```python
from build123d import *

# Parameters (mm, degrees)
SKETCH_1_R               = 2.5
EXTRUDE_1_DEPTH          = 2.5
CUT_EXTRUDE_1_REACH      = 65.602
SKETCH_2_R               = 2
PATTERN_CIRCULAR_1_COUNT = 6
FILLET_1_R               = 3


with BuildPart() as part:
    # 草圖1 → 填料-伸長1 (new, symmetric)
    with BuildSketch(Plane.XY):
        with BuildLine():
            Line((17.895530168, 10), (50, 10))
            ThreePointArc((50, 10), (60, 0), (50, -10))
            Line((50, -10), (17.895530168, -10))
            ThreePointArc((17.895530168, -10), (-20.5, 0), (17.895530168, 10))
        make_face()
        with Locations((50, 0)):
            Circle(SKETCH_1_R, mode=Mode.SUBTRACT)
    extrude(amount=EXTRUDE_1_DEPTH, both=True)

    # 草圖2 → 除料-伸長1 (cut, up to next)
    with BuildSketch(Plane.XY.offset(2.5), mode=Mode.PRIVATE) as cut_extrude_1_sk1:
        with Locations((0, 15.5)):
            Circle(SKETCH_2_R)
    cut_extrude_1_tool1 = extrude(cut_extrude_1_sk1.sketch, amount=-CUT_EXTRUDE_1_REACH, mode=Mode.PRIVATE) & part.part
    cut_extrude_1 = cut_extrude_1_tool1.solids().sort_by_distance((0, 15.5, 2.5))[0]
    add(cut_extrude_1, mode=Mode.SUBTRACT)

    # 環狀複製排列1: 除料-伸長1 ×6 about axis
    pattern_circular_1_axis = Axis((0, 0, 0), (0, 0, 1))
    for i in range(1, PATTERN_CIRCULAR_1_COUNT):
        add(cut_extrude_1.rotate(pattern_circular_1_axis, i * 360 / PATTERN_CIRCULAR_1_COUNT), mode=Mode.SUBTRACT)

    # 圓角1
    fillet_1_edges = [part.edges().sort_by_distance(p)[0] for p in [
        (17.895530168, 10, 0),
        (17.895530168, -10, 0),
    ]]
    fillet(fillet_1_edges, radius=FILLET_1_R)


solid = part.part
```
Verification items for the finished model (mm, model axes). A direction names the side the tool comes from. Round coordinates to 2 decimals unless told otherwise and drop trailing zeros. Write each loop counter-clockwise with the first axis right and the second up, starting at its lowest first coordinate (ties: lowest second). Pieces come first, ordered by that corner, then holes.
1. Section check B-B on x = 0. Enter the section's corners in (y, z).
2. Section check C-C on z = 0.65. Enter the section's corners in (x, y).
3. Draft check along Y on faces 1 (the cylindrical face through (52.31, -0.96, -0.04)), 2 (the cylindrical face through (18.141, -10.366, 0.035)), 3 (the cylindrical face through (60, 0, 0)). Enter one of: +Y half, -Y half, draft (parallel to the pull), parting line (faces both ways), or undercut.
4. Access from +Z, -Z, +X, -X, +Y, -Y to the whole of each face (thin tool, end or side, straight path). Record for faces 4 (the flat face through (35, -10, 0)), 5 (the cylindrical face through (-13.86, -9.7, 0.04)), 6 (the flat face through (35, 10, 0)).
5. Section check D-D on y = 7.75. Enter the section's corners in (x, z).
6. Scan lines: L1, parallel to Y at x = 0, z = 1.4; L2, parallel to X at y = 9, z = 1.8; L3, parallel to X at y = 8, z = -0.2. Record each from-to range of solid material in increasing order.
7. Section check A-A on y = 0. Enter the section's corners in (x, z).
Answer:
1. outline: (-20.5, -2.5) - (-17.5, -2.5) - (-17.5, 2.5) - (-20.5, 2.5) - close; (-13.5, -2.5) - (13.5, -2.5) - (13.5, 2.5) - (-13.5, 2.5) - close; (17.5, -2.5) - (20.5, -2.5) - (20.5, 2.5) - (17.5, 2.5) - close
2. outline: (17.08, -11.34) arc R3 cw to (19.58, -10) - (50, -10) arc R10 ccw to (50, 10) - (19.58, 10) arc R3 cw to (17.08, 11.34) arc R20.5 ccw (long way) to start; hole circle Ø4 at (-13.42, -7.75); hole circle Ø4 at (-13.42, 7.75); hole circle Ø4 at (0, -15.5); hole circle Ø4 at (0, 15.5); hole circle Ø4 at (13.42, -7.75); hole circle Ø4 at (13.42, 7.75); hole circle Ø5 at (50, 0)
3. face 1: undercut
3. face 2: -Y half
3. face 3: parting line
4. face 4: +Z, -Z, +X, -Y
4. face 5: +Z, -Z
4. face 6: +Z, -Z, +X, +Y
5. outline: (-18.98, -2.5) - (-15.42, -2.5) - (-15.42, 2.5) - (-18.98, 2.5) - close; (-11.42, -2.5) - (11.42, -2.5) - (11.42, 2.5) - (-11.42, 2.5) - close; (15.42, -2.5) - (56.32, -2.5) - (56.32, 2.5) - (15.42, 2.5) - close
6. L1: y = -20.5 to -17.5, -13.5 to 13.5, 17.5 to 20.5
6. L2: x = -18.42 to -14.98, -11.86 to 11.86, 14.98 to 54.36
6. L3: x = -18.87 to -15.41, -11.44 to 11.44, 15.41 to 56
7. outline: (-20.5, -2.5) - (47.5, -2.5) - (47.5, 2.5) - (-20.5, 2.5) - close; (52.5, -2.5) - (60, -2.5) - (60, 2.5) - (52.5, 2.5) - close
